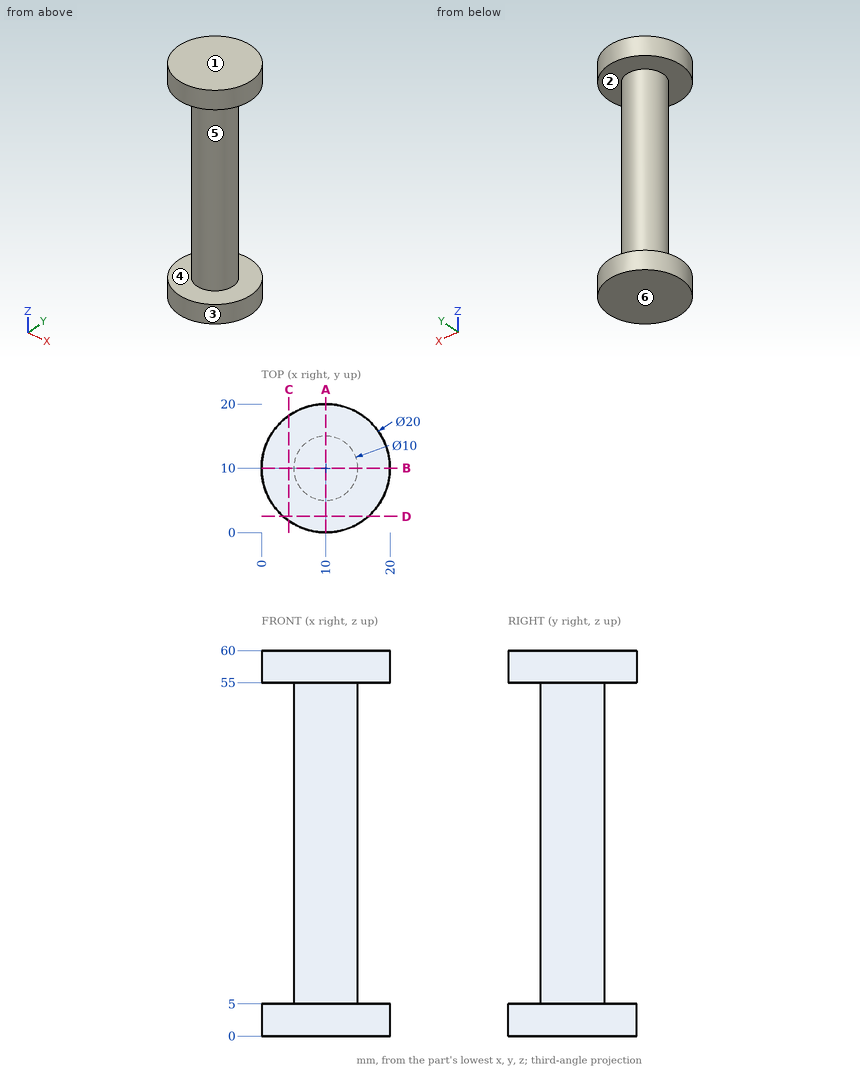
Here's the drawing with two shaded views (mm, measured from the low corner). I have some questions. A direction names the side the tool comes from. Coordinates: 2 decimals unless noted, no trailing zeros. Loops run counter-clockwise (first coordinate to the right, second up) from the corner with the lowest first, then second, coordinate; pieces in that order, holes last. Notation, with made-up numbers: (-10, 32) -> (44, 32) arc R17 ccw to (44, 47) -> close; hole circle Ø10 at (54, 6). An arc over 180 degrees is marked (long way). Answer as a JSON object with one key per item and string values.
1) Imagine slicing it at D-D (y = 2.5). Please give me the cut outline in (x, z).
Results:
{"outline": "(3.39, 0) -> (16.61, 0) -> (16.61, 5) -> (3.39, 5) -> close; (3.39, 55) -> (16.61, 55) -> (16.61, 60) -> (3.39, 60) -> close"}
2) For P1, Ø2, axis at x = 15.5, z = 15, coming from the -Y side; P2, Ø10, axis at y = 15, z = 17.5, coming from the +X side; P3, Ø1.5, axis at x = 5, z = 26.5, coming from the -Y side, each with a flat end and sliding along its axis, tell me the tip position at first contact or that it passes through.
Results:
{"P1": "stops at y = 7.82", "P2": "stops at x = 15", "P3": "stops at y = 7.37"}
3) Thinking about a two-plate mould opening in Z: for the marked faces 1, 2, 3 and 4, which applies, pulls with the +Z half, pulls with the -Z half, needs draft (parallel to the pull), parting line crosses it, or undercut?
Results:
{"face 1": "pulls with the +Z half", "face 2": "undercut", "face 3": "needs draft", "face 4": "undercut"}
4) If I drill on line 1 (Z direction, x = 15.25, y = 15.75); line 2 (X direction, y = 6.25, z = 31.5); line 3 (Y direction, x = 8.5, z = 22.5), over which ranges is the centre line in solid material (lowest first)?
Results:
{"line 1": "z = 0 to 5, 55 to 60", "line 2": "x = 6.69 to 13.31", "line 3": "y = 5.23 to 14.77"}
5) For the marked faces 5 and 6, which set-ups out of +Z, -Z, +X, -X, +Y, -Y let a thin tool reach every point of the face, with its end or its side?
Results:
{"face 5": "none", "face 6": "-Z, +X, -X, +Y, -Y"}
6) Imagine slicing it at A-A (x = 10). Please give me the cut outline in (y, z).
Results:
{"outline": "(0, 0) -> (20, 0) -> (20, 5) -> (15, 5) -> (15, 55) -> (20, 55) -> (20, 60) -> (0, 60) -> (0, 55) -> (5, 55) -> (5, 5) -> (0, 5) -> close"}
7) Imagine slicing it at C-C (x = 4.25). Please give me the cut outline in (y, z).
Results:
{"outline": "(1.82, 0) -> (18.18, 0) -> (18.18, 5) -> (1.82, 5) -> close; (1.82, 55) -> (18.18, 55) -> (18.18, 60) -> (1.82, 60) -> close"}
